Autodesk Inventor part; units mm, degrees
ref_plane "YZ Plane" through (0, 0, 0) normal (1, 0, 0) x (0, 1, 0)
ref_plane "XZ Plane" through (0, 0, 0) normal (0, 1, 0) x (-1, 0, 0)
ref_plane "XY Plane" through (0, 0, 0) normal (0, 0, 1) x (1, 0, 0)
sketch "Sketch1" plane through (0, 0, 0) normal (0, 0, 1) x (1, 0, 0)
  circle A0 centre (0, 0) radius 52
  circle A1 centre (0, 0) radius 17.45
  circle A2 centre (0, 0) radius 40 construction
  circle A3 centre (40, 0) radius 5.5
  circle A4 centre (28.2843, 28.2843) radius 5.5
  circle A5 centre (0, 40) radius 5.5
  circle A6 centre (-28.2843, 28.2843) radius 5.5
  circle A7 centre (-40, 0) radius 5.5
  circle A8 centre (-28.2843, -28.2843) radius 5.5
  circle A9 centre (0, -40) radius 5.5
  circle A10 centre (28.2843, -28.2843) radius 5.5
  dimension "d39" = 80
  dimension "d31" = 34.9
  dimension "d32" = 104
  dimension "d40" = 11
  dimension "d43" = 360
extrude "Plate1" add sketch "Sketch1" against normal blind 2
equation "\"d15\" = Thickness"
equation "\"BendRadius\" = Thickness"
equation "\"BendReliefWidth\" = Thickness"
equation "\"BendReliefDepth\" = 0.5 * Thickness"
equation "\"CornerReliefSize\" = 4 * Thickness"
equation "\"MinimumRemnant\" = 2 * Thickness"
equation "\"TransitionRadius\" = BendRadius"
equation "\"JacobiRadiusSize\" = BendRadius"
equation "\"GapSize\" = Thickness"
properties part number "DMF flange small gear 2"
The listing builds one solid part. Answer for the finished solid, in the listing's coordinates (mm). Coordinates: 2 decimals unless noted, no trailing zeros. Write each loop counter-clockwise with the first axis right and the second up, starting at its lowest first coordinate (ties: lowest second). Pieces come first, ordered by that corner, then holes. Notation, with made-up numbers: (34, 86) -> (63, 86) arc R19 ccw to (63, 91) -> close; hole circle Ø7 at (10.25, 61). An arc over 180 degrees is marked (long way). One line per question, with ' | ' between items.
1. Given pin 1 Ø17.5 at (x, y) = (28.28, -28.28) entering from -Z; pin 2 Ø1 at (y, z) = (24, -1.5) entering from -X, each flat-ended and moving along its own axis, determine where each tip first touches the part or whether it passes through.
Verdict:
pin 1: stops at z = -2 | pin 2: stops at x = -46.39
2. Straight lines are drawn through the part: line 1 (X direction, y = 24, z = -0.45); line 2 (Y direction, x = 30.5, z = -0.6); line 3 (Y direction, x = -24.5, z = -1.75). For each, find the intervals that lie inside material, in ascending order.
Verdict:
line 1: x = -46.13 to -31.73, -24.84 to 24.84, 31.73 to 46.13 | line 2: y = -42.12 to -33.32, -23.25 to 23.25, 33.32 to 42.12 | line 3: y = -45.87 to -32.28, -24.29 to 24.29, 32.28 to 45.87
3. Section B-B (y = 37) is taken. Determine the outline of the cut face in (x, z).
Verdict:
outline: (-36.54, -2) -> (-4.61, -2) -> (-4.61, 0) -> (-36.54, 0) -> close; (4.61, -2) -> (36.54, -2) -> (36.54, 0) -> (4.61, 0) -> close
4. Section A-A (x = 0) is taken. Determine the outline of the cut face in (y, z).
Verdict:
outline: (-52, -2) -> (-45.5, -2) -> (-45.5, 0) -> (-52, 0) -> close; (-34.5, -2) -> (-17.45, -2) -> (-17.45, 0) -> (-34.5, 0) -> close; (17.45, -2) -> (34.5, -2) -> (34.5, 0) -> (17.45, 0) -> close; (45.5, -2) -> (52, -2) -> (52, 0) -> (45.5, 0) -> close
5. For a pull along Y with two mould halves and no side action, classify faces 1 (the cylindrical face through (-41.265, -31.641, -0.986)), 2 (the cylindrical face through (-0.716, 45.453, -0.986)), 3 (the flat face through (22, 1, -2)) as released by +Y, released by -Y, zero draft, split by the parting line, or undercut.
Verdict:
face 1: split by the parting line | face 2: undercut | face 3: zero draft
6. Section D-D (z = -1.1) is taken. State how many separate pieces and enclosed holes the cut face has, and give its area (3 significant figures).
Verdict:
separate pieces: 1 | enclosed holes: 9 | area: 6,780 mm^2
7. Section C-C (x = -40.5) is taken. Determine the outline of the cut face in (y, z).
Verdict:
outline: (-32.62, -2) -> (-5.48, -2) -> (-5.48, 0) -> (-32.62, 0) -> close; (5.48, -2) -> (32.62, -2) -> (32.62, 0) -> (5.48, 0) -> close
